from build123d import *

# Parameters (mm, degrees)
CROQUIS1_R              = 6
SALIENTE_EXTRUIR1_DEPTH = 400
CROQUIS2_OUTSIDE_W      = 94.072
CROQUIS2_OUTSIDE_H      = 94.072
CROQUIS2_OUTSIDE_R      = 4
CORTAR_EXTRUIR3_DEPTH   = 40
CROQUIS3_R              = 4
SALIENTE_EXTRUIR2_DEPTH = 40


with BuildPart() as part:
    # Croquis1 → Saliente-Extruir1 (new body)
    with BuildSketch(Plane.XY):
        Circle(CROQUIS1_R)
    extrude(amount=SALIENTE_EXTRUIR1_DEPTH)

    # Croquis2 outside → Cortar-Extruir3 (cut)
    with BuildSketch(Plane.XY.offset(400)):
        Rectangle(CROQUIS2_OUTSIDE_W, CROQUIS2_OUTSIDE_H)
        Circle(CROQUIS2_OUTSIDE_R, mode=Mode.SUBTRACT)
    extrude(amount=-CORTAR_EXTRUIR3_DEPTH, mode=Mode.SUBTRACT)

    # Croquis3 → Saliente-Extruir2 (add)
    with BuildSketch(Plane(origin=(0, 0, 0), x_dir=(-1, 0, 0), z_dir=(0, 0, -1))):
        with Locations(Location((0, 0, 0), (0, 0, 180))):
            Circle(CROQUIS3_R)
    extrude(amount=SALIENTE_EXTRUIR2_DEPTH)


solid = part.part
The model under review builds one solid part; all positions refer to its coordinate system, in mm. A direction names the side the tool comes from. Give positions to 0.01 mm unless a question says otherwise; leave off trailing zeros. Write each loop counter-clockwise with the first axis right and the second up, starting at its lowest first coordinate (ties: lowest second). Pieces come first, ordered by that corner, then holes.
1. Add section C-C, the plane z = 126. Write out the cut boundary in (x, y).
2. Wall thickness on L1, parallel to Z at x = 2.75, y = -4.75; L2, parallel to X at y = 4.5, z = 294; L3, parallel to Y at x = -0.5, z = 185: over which ranges is each line inside the solid? List them lowest first.
3. Add section A-A, the plane y = 0. Write out the cut boundary in (x, z).
4. Tool access review of faces 1 (the flat face through (-1.42, -3.92, 0)), 2 (the flat face through (-1.42, -3.92, 360)), 3 (the flat face through (0, 0, 400)): name each direction out of +Z, -Z, +X, -X, +Y, -Y from which nothing blocks a thin tool from reaching the whole face with its end or side.
5. For P1, Ø1, axis at y = 2.5, z = 67.5, coming from the -X side; P2, Ø1, axis at x = -4, z = 115, coming from the +Y side, all flat-tipped, find the tip position at first contact; note any pin that passes through.
Worked answers:
1. outline: circle Ø12 at (0, 0)
2. L1: z = 0 to 360
2. L2: x = -3.97 to 3.97
2. L3: y = -5.98 to 5.98
3. outline: (-6, 0) - (-4, 0) - (-4, -40) - (4, -40) - (4, 0) - (6, 0) - (6, 360) - (4, 360) - (4, 400) - (-4, 400) - (-4, 360) - (-6, 360) - close
4. face 1: -Z
4. face 2: +Z
4. face 3: +Z, +X, -X, +Y, -Y
5. P1: stops at x = -5.66
5. P2: stops at y = 4.87
